Solid Edge part; units mm, degrees
sketch "Sketch1" plane through (0, 0, 0) normal (0, 0, 1) x (1, 0, 0)
  circle A0 centre (0, 0) radius 10
extrude "Protrusion1" add sketch "Sketch1" along normal blind 600
sketch "Sketch2" plane through (0, 0, 0) normal (0, 0, -1) x (1, 0, 0)
  circle A0 centre (0, 0) radius 6
extrude "ExtrudedProtrusion_2" add sketch "Sketch2" along normal mid plane 35
cosmetic_thread "Thread1"
sketch "Sketch3" plane through (0, 0, 600) normal (0, 0, 1) x (0, 1, 0)
  circle A0 centre (0, 0) radius 6
extrude "ExtrudedProtrusion_3" add sketch "Sketch3" along normal blind 25
cosmetic_thread "Thread2"
sketch "Sketch4" plane through (0, -10, 250) normal (0, -1, 0) x (0, 0, -1)
  line L0 (158, -2) -> (150, -2)
  line L1 (150, -2) -> (150, 2)
  line L2 (150, 2) -> (158, 2)
  line L3 (158, 2) -> (158, -2)
  dimension "D1" = 158
  dimension "D2" = 150
extrude "ExtrudedCutout_5" cut sketch "Sketch4" against normal blind 2
sketch "Sketch5" plane through (0, 0, 0) normal (1, 0, 0) x (0, 1, 0)
  line L0 (-10, 100) -> (-9, 100)
  line L1 (-9, 100) -> (-9, 101)
  line L2 (-9, 101) -> (-10, 101)
  line L3 (-10, 101) -> (-10, 100)
  dimension "D1" = 10
  dimension "D2" = 10
revolve "RevolvedCutout1" cut sketch "Sketch5" angle 360 about axis through (0, 0, -57) along (0, 0, 1)
properties material "Steel"
Geometry check sheet. Reference: the model listing, model coordinates, mm. A direction names the side the tool comes from. Give positions to 0.01 mm unless a question says otherwise; leave off trailing zeros. Order: outer loops, then holes, each group sorted by start corner. A loop starts at its lowest first (then second) coordinate and runs counter-clockwise, first axis right, second up. Notation, with made-up numbers: (-13.75, -28) - (44.25, -28) arc R20 cw to (44.25, -9) - close; hole circle Ø4 at (85, 36). An arc over 180 degrees is marked (long way). Answer in a Markdown table with one row per item. Add a question column.
Q1. Gauge pin test, flat ends, axial feed: pin 1 (0.5 mm diameter, centred on y = -9, z = 96.5, fed in from +X); pin 2 (6 mm diameter, centred on y = 6, z = 510.5, fed in from -X); pin 3 (1 mm diameter, centred on y = 4, z = 208.5, fed in from +X). Record the tip position at first contact, or that the pin passes through.
Q2. Tool access check on faces 5 (the cylindrical face through (-6, 0, -9)), 6 (the cylindrical face through (-2.17, 9.76, 347.01)), 7 (the flat face through (0, 0, 625)), 8 (the cylindrical face through (0, -6, 612)), 9 (the flat face through (2, 9, 100)). Record the directions out of +Z, -Z, +X, -X, +Y, -Y that give a thin tool (end or side, any length) a straight path to the whole face; none if there is none.
Q3. Mould release check, pull along Z, two halves, no side actions. Record for faces 1 (the flat face through (7, 0, 0)), 2 (the flat face through (7, 0, 600)), 3 (the cylindrical face through (-2.17, 9.76, 49.3)), 4 (the cylindrical face through (8.923, 1.172, 100.507)): pulls with the +Z half, pulls with the -Z half, needs draft (parallel to the pull), parting line crosses it, or undercut.
Q4. Cross-section at A-A, the plane y = 0. Enter the section's corners in (x, z), then the cut area to 3 significant figures.
Q5. Material ranges on probe 1 along Z at (x, y) = (2, 9); probe 2 along X at (y, z) = (-4.5, 369.5); probe 3 along Y at (x, z) = (0, 186), recorded low to high. Write a range as from..to.
Q6. Cross-section at B-B, the plane z = 278. Enter the section's corners in (x, y).
Check values:
| question | item | result |
|---|---|---|
| 1 | pin 1 | stops at x = 4.84 |
| 1 | pin 2 | stops at x = -9.54 |
| 1 | pin 3 | stops at x = 9.37 |
| 2 | face 5 | -Z |
| 2 | face 6 | +Z, -Z |
| 2 | face 7 | +Z, +X, -X, +Y, -Y |
| 2 | face 8 | +Z |
| 2 | face 9 | none |
| 3 | face 1 | pulls with the -Z half |
| 3 | face 2 | pulls with the +Z half |
| 3 | face 3 | needs draft |
| 3 | face 4 | undercut |
| 4 | outline | (-10, 0) - (-6, 0) - (-6, -17.5) - (6, -17.5) - (6, 0) - (10, 0) - (10, 100) - (9, 100) - (9, 101) - (10, 101) - (10, 600) - (6, 600) - (6, 625) - (-6, 625) - (-6, 600) - (-10, 600) - (-10, 101) - (-9, 101) - (-9, 100) - (-10, 100) - close |
| 4 | area | 12,500 mm^2 |
| 5 | probe 1 | z = 0..100, 101..600 |
| 5 | probe 2 | x = -8.93..8.93 |
| 5 | probe 3 | y = -10..10 |
| 6 | outline | circle Ø20 at (0, 0) |
